Verification items for the finished model (mm, model axes). A direction names the side the tool comes from. Coordinates: 2 decimals unless noted, no trailing zeros. Order: outer loops, then holes, each group sorted by start corner. A loop starts at its lowest first (then second) coordinate and runs counter-clockwise, first axis right, second up. Notation, with made-up numbers: (14.25, 23.5) -> (54.25, 23.5) arc R8 ccw to (54.25, 37.5) -> close; hole circle Ø10 at (46.25, -33). An arc over 180 degrees is marked (long way). Use CSV: the item, a comma, the result in double quotes. Start each with the question number.
1) Scan lines: line 1 along Y through (x, z) = (0, 89.25); line 2 along X through (y, z) = (-177, 98.5); line 3 along Y through (x, z) = (-31, 91). Record each from-to range of solid material in increasing order.
2) Tool access check on faces 4 (the cylindrical face through (-32.743, -188.716, 94.084)), 5 (the flat face through (-25.789, -175.535, 94.084)), 6 (the flat face through (33, -230, 88)). Record the directions out of +Z, -Z, +X, -X, +Y, -Y that give a thin tool (end or side, any length) a straight path to the whole face; none if there is none.
3) Sectioned sample at B-B on y = -215.5. Give the number of separate pieces and of enclosed holes in the cut face, then the cut area to 3 significant figures.
4) Sectioned sample at A-A on z = 87. Record the boundary of the cut face in (x, y), then the cut area to 3 significant figures.
5) Go/stop test with flat-tipped pins: pin 1 (6.5 mm diameter, centred on x = -31, y = -239, fed in from -Z); pin 2 (4 mm diameter, centred on x = 0, y = -193, fed in from +Z). Record where each tip stops, or that it passes through.
6) Release check for a two-part mould opening along Y. For faces 1 (the cylindrical face through (32.743, -227.284, 94.084)), 2 (the flat face through (0, -173, 94)), 3 (the flat face through (-35, -208, 94)) record: released by +Y, released by -Y, zero draft, split by the parting line, or undercut.
from build123d import *

# Parameters (mm, degrees)
SKETCH030_W           = 70
SKETCH030_H           = 70
SKETCH030_R           = 2.1
PAD019_DEPTH          = 10
POCKET014_DEPTH       = 221.9910987672
POLARPATTERN002_COUNT = 4
FILLET011_R           = 4
SKETCH032_R           = 34
POCKET018_DEPTH       = 18.5
POCKET017_DEPTH       = 6
POLARPATTERN003_COUNT = 4


with BuildPart() as part:
    # Sketch030 → Pad019 (new body, symmetric)
    with BuildSketch(Plane.XY):
        Rectangle(SKETCH030_W, SKETCH030_H)
        with Locations((-31, 31)):
            Circle(SKETCH030_R, mode=Mode.SUBTRACT)
        with Locations((31, 31)):
            Circle(SKETCH030_R, mode=Mode.SUBTRACT)
        with Locations((31, -31)):
            Circle(SKETCH030_R, mode=Mode.SUBTRACT)
        with Locations((-31, -31)):
            Circle(SKETCH030_R, mode=Mode.SUBTRACT)
    extrude(amount=PAD019_DEPTH, both=True)

    # Sketch029 (on Face10 of Pad019) → Pocket014 (cut, through all)
    with BuildSketch(Plane.XY.offset(10)):
        with BuildLine():
            ThreePointArc((-8.7274847969, 32.8607822354), (-28.4137092085, 18.6724698156), (-33.6262546007, -5.0274249403))
            add(Edge.make_bspline(
                [(6.6856437151, 14.5362363807), (-9.201321, 21.706085), (-33.6262546007, -5.0274249403)],
                knots=[0, 0, 0, 1, 1, 1], degree=2))
            add(Edge.make_bspline(
                [(6.6856437151, 14.5362363807), (-1.353872, 27.495132), (-8.7274847969, 32.8607822354)],
                knots=[0, 0, 0, 1, 1, 1], degree=2))
        make_face()
    pocket014 = extrude(amount=-POCKET014_DEPTH, mode=Mode.SUBTRACT)

    # PolarPattern002: Pocket014 ×4 about axis
    polarpattern002_axis = Axis((0, 0, 10), (0, 0, 1))
    for i in range(1, POLARPATTERN002_COUNT):
        add(pocket014.rotate(polarpattern002_axis, i * 360 / POLARPATTERN002_COUNT), mode=Mode.SUBTRACT)

    # Fillet011
    fillet011_edges = [part.edges().sort_by_distance(p)[0] for p in [
        (35, 35, 0),
        (-35, 35, 0),
        (35, -35, 0),
        (-35, -35, 0),
    ]]
    fillet(fillet011_edges, radius=FILLET011_R)

    # Sketch032 (on Face5 of Fillet011) → Pocket018 (cut)
    with BuildSketch(Plane.XY.offset(10)):
        Circle(SKETCH032_R)
    extrude(amount=-POCKET018_DEPTH, mode=Mode.SUBTRACT)

    # Sketch033 → Pocket017 (cut, symmetric)
    with BuildSketch(Plane.XY):
        with BuildLine():
            ThreePointArc((23.3238075794, 30), (0, 38), (-23.3238075794, 30))
            Line((-23.3238075794, 30), (-29, 35.6761924206))
            Line((-29, 35.6761924206), (-29, 47.6761924206))
            Line((-29, 47.6761924206), (29, 47.6761924206))
            Line((29, 47.6761924206), (29, 35.6761924206))
            Line((29, 35.6761924206), (23.3238075794, 30))
        make_face()
    pocket017 = extrude(amount=POCKET017_DEPTH, both=True, mode=Mode.SUBTRACT)

    # PolarPattern003: Pocket017 ×4 about axis
    polarpattern003_axis = Axis((0, 0, 0), (0, 0, 1))
    for i in range(1, POLARPATTERN003_COUNT):
        add(pocket017.rotate(polarpattern003_axis, i * 360 / POLARPATTERN003_COUNT), mode=Mode.SUBTRACT)


with BuildPart() as part_1:
    # Body013 placement: moved
    add(part.part.moved(Location((0, -208, 94))))


solid = part_1.part
Answers follow:
1,line 1,"y = -243 to -242, -174 to -173"
1,line 2,"x = -35 to -33.1, -28.9 to -24.32, -21.98 to -13.96, 13.96 to 21.98, 24.32 to 28.9, 33.1 to 35"
1,line 3,"y = -243 to -241.1, -236.9 to -232.32, -229.98 to -221.96, -194.04 to -186.02, -183.68 to -179.1, -174.9 to -173"
2,face 4,"-X"
2,face 5,"+Y"
2,face 6,"+X"
3,separate pieces,"3"
3,enclosed holes,"0"
3,area,"128 mm²"
4,outline,"(-35, -239) arc R4 ccw to (-31, -243) -> (31, -243) arc R4 ccw to (35, -239) -> (35, -177) arc R4 ccw to (31, -173) -> (-31, -173) arc R4 ccw to (-35, -177) -> close; hole circle Ø68 at (0, -208); hole circle Ø4.2 at (-31, -239); hole circle Ø4.2 at (-31, -177); hole circle Ø4.2 at (31, -239); hole circle Ø4.2 at (31, -177)"
4,area,"1,200 mm²"
5,pin 1,"stops at z = 84"
5,pin 2,"stops at z = 85.5"
6,face 1,"undercut"
6,face 2,"released by +Y"
6,face 3,"zero draft"
